The model under review builds one solid part; all positions refer to its coordinate system, in mm. A direction names the side the tool comes from. Round coordinates to 2 decimals unless told otherwise and drop trailing zeros. One line per item, written item: value. Start each with the question number.
1) For P1, Ø1, axis at y = -99.5, z = 0.5, coming from the -X side; P2, Ø1.8, axis at x = -173.5, y = -155.5, coming from the +Z side; P3, Ø1.8, axis at x = -54.5, y = -154, coming from the +Z side; P4, Ø2.5, axis at x = -150.5, y = -150.5, coming from the +Z side, all flat-tipped, find the tip position at first contact; note any pin that passes through.
2) Tool access review of faces 5 (the face through (-114, -41.59, 1)), 6 (the face through (-76, -152, 2.5)): name each direction out of +Z, -Z, +X, -X, +Y, -Y from which nothing blocks a thin tool from reaching the whole face with its end or side.
3) Wall thickness on probe 1 along X at (y, z) = (-155, 2.3); probe 2 along X at (y, z) = (-102, 1.15); probe 3 along X at (y, z) = (-52, 1.4): over which ranges is each line inside the solid? List them lowest first.
4) Mouldability with a two-part tool opening along X and no side actions: class faces 1 (the face through (-58.23, -154.96, 2.01)), 2 (the face through (-115, -101, 3)), 3 (the face through (-56.6, -49.1, 1.5)), 4 (the face through (-52.16, -44.69, 1.48)) as +X half, -X half, draft (parallel to the pull), parting line (faces both ways), or undercut.
from build123d import *

# Parameters (mm, degrees)
SKIZZE1_R                       = 1.7
AUFSATZ_LINEAR_AUSTRAGEN1_DEPTH = 3
SKIZZE2_R                       = 3
SCHNITT_LINEAR_AUSTRAGEN1_DEPTH = 2
SKIZZE3_R                       = 4
SCHNITT_LINEAR_AUSTRAGEN2_DEPTH = 0.5


with BuildPart() as part:
    # Skizze1 → Aufsatz-Linear austragen1 (new body)
    with BuildSketch(Plane.XY):
        with BuildLine():
            Line((-49.2275, -151.2967), (-49.2275, -51.8905))
            ThreePointArc((-49.2275, -51.8905), (-52.244300154, -44.607300154), (-59.5275, -41.5905))
            Line((-59.5275, -41.5905), (-169.0581, -41.5905))
            ThreePointArc((-169.0581, -41.5905), (-176.514207067, -44.783915623), (-179.34742314, -52.3842))
            Line((-179.34742314, -52.3842), (-179.34742314, -150.803560266))
            ThreePointArc((-179.34742314, -150.803560266), (-176.514004305, -158.403485592), (-169.0581, -161.5967))
            Line((-169.0581, -161.5967), (-59.5275, -161.5967))
            ThreePointArc((-59.5275, -161.5967), (-52.244300154, -158.579899846), (-49.2275, -151.2967))
        make_face()
        with Locations((-172.84742314, -155.0967)):
            Circle(SKIZZE1_R, mode=Mode.SUBTRACT)
        with Locations((-55.2338, -155.0967)):
            Circle(SKIZZE1_R, mode=Mode.SUBTRACT)
        with Locations((-55.2338, -48.0905)):
            Circle(SKIZZE1_R, mode=Mode.SUBTRACT)
        with Locations((-172.84742314, -48.0905)):
            Circle(SKIZZE1_R, mode=Mode.SUBTRACT)
    extrude(amount=AUFSATZ_LINEAR_AUSTRAGEN1_DEPTH)

    # Skizze2 → Schnitt-Linear austragen1 (cut)
    with BuildSketch(Plane.XY.offset(3)):
        with Locations((-172.84742314, -155.0967)):
            Circle(SKIZZE2_R)
        with Locations((-55.2338, -155.0967)):
            Circle(SKIZZE2_R)
    extrude(amount=-SCHNITT_LINEAR_AUSTRAGEN1_DEPTH, mode=Mode.SUBTRACT)

    # Skizze3 → Schnitt-Linear austragen2 (cut)
    with BuildSketch(Plane.XY.offset(3)):
        with Locations((-152.34742314, -151.5967)):
            Circle(SKIZZE3_R)
        with Locations(Location((-76.23817686, -151.5967, 0), (0, 0, 180))):
            Circle(SKIZZE3_R)
    extrude(amount=-SCHNITT_LINEAR_AUSTRAGEN2_DEPTH, mode=Mode.SUBTRACT)


solid = part.part
Checked values:
1. P1: stops at x = -179.35
1. P2: passes through
1. P3: stops at z = 1
1. P4: stops at z = 2.5
2. face 5: +Z, -Z, +X, -X, +Y
2. face 6: +Z
3. probe 1: x = -178.67 to -175.85, -169.85 to -58.23, -52.24 to -49.92
3. probe 2: x = -179.35 to -49.23
3. probe 3: x = -179.36 to -49.23
4. face 1: undercut
4. face 2: draft
4. face 3: undercut
4. face 4: +X half
